Source: three-view drawing plus pictorial views. Frame: mm from the lowest corner of the part. A direction names the side the tool comes from. Give positions to 0.01 mm unless a question says otherwise; leave off trailing zeros. Order: outer loops, then holes, each group sorted by start corner. A loop starts at its lowest first (then second) coordinate and runs counter-clockwise, first axis right, second up.
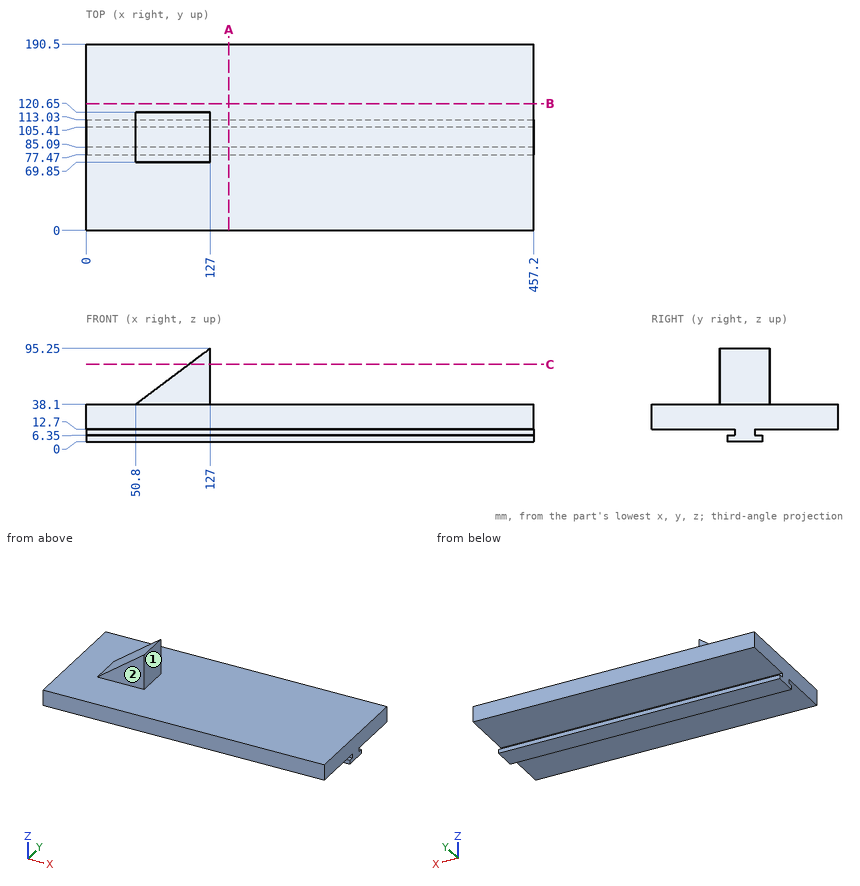
(1) Section C-C, the plane z = 79. Return loops of the section in (x, y).
(2) Access query for the marked faces 1 and 2. Directions: +Z, -Z, +X, -X, +Y, -Y. A direction counts if a zero-diameter tool reaches every point of the face in a straight line with its end or side. Return the directions, or none.
(3) Section A-A, the plane x = 146. Return loops of the section in (y, z), plus the area to 3 significant figures.
(4) Pin query (flat end, axial travel): pin 1 Ø8 at (x, y) = (83, 38) entering from +Z; pin 2 Ø10 at (y, z) = (124.5, 59.5) entering from +X; pin 3 Ø5 at (x, z) = (226.5, 8) entering from +Y. Return the tip coordinate at first contact, or that it passes through.
(5) Section B-B, the plane y = 129.5. Return loops of the section in (x, z), plus the area to 3 significant figures.
(6) Line query: line 1 along Z through (x, y) = (284, 11.5); line 2 along Y through (x, z) = (124.5, 78.5); line 3 along X through (y, z) = (74, 45). Output: solid intervals per line, ascending.
Checks:
1. outline: (105.33, 69.85) - (127, 69.85) - (127, 120.65) - (105.33, 120.65) - close
2. face 1: +Z, +X, +Y, -Y
2. face 2: +Z, +X, -X, -Y
3. outline: (0, 12.7) - (85.09, 12.7) - (85.09, 6.35) - (77.47, 6.35) - (77.47, 0) - (113.03, 0) - (113.03, 6.35) - (105.41, 6.35) - (105.41, 12.7) - (190.5, 12.7) - (190.5, 38.1) - (0, 38.1) - close
3. area: 5,190 mm2
4. pin 1: stops at z = 38.1
4. pin 2: stops at x = 127
4. pin 3: stops at y = 113.03
5. outline: (0, 12.7) - (457.2, 12.7) - (457.2, 38.1) - (0, 38.1) - close
5. area: 11,600 mm2
6. line 1: z = 12.7 to 38.1
6. line 2: y = 69.85 to 120.65
6. line 3: x = 60 to 127
